Geometry check sheet. Reference: the model listing, model coordinates, mm. Give positions to 0.01 mm unless a question says otherwise; leave off trailing zeros. Order: outer loops, then holes, each group sorted by start corner. A loop starts at its lowest first (then second) coordinate and runs counter-clockwise, first axis right, second up. Notation, with made-up numbers: M -4,-32.5 L 11,-32.5 A32 cw 11,-1.5 Z; hole C 0.25,-31.75 d2. An arc over 180 degrees is marked long. Put each result on its own line as item: value. Start each with the question number.
Q1. Section check A-A on x = 0. Record the cut outline in (y, z) (3 decimals).
Q2. Section check C-C on x = -36. Record the cut outline in (y, z) (3 decimals).
Q3. Material ranges on L1, parallel to Z at x = -39, y = -72 (3 decimals); L2, parallel to Y at x = 17, z = -2; L3, parallel to Y at x = -4, z = -1.75, recorded low to high.
Q4. Section check D-D on y = -52. Record the cut outline in (x, z) (3 decimals), then the cut area to 3 significant figures.
Q5. Go/stop test with flat-tipped pins: pin 1 (2 mm diameter, centred on y = 0, z = 0, fed in from +X); pin 2 (3 mm diameter, centred on y = 72, z = 0, fed in from -X). Record where each tip stops, or that it passes through.
Q6. Section check B-B on y = 23.5. Record the cut outline in (x, z) (3 decimals), then the cut area to 3 significant figures.
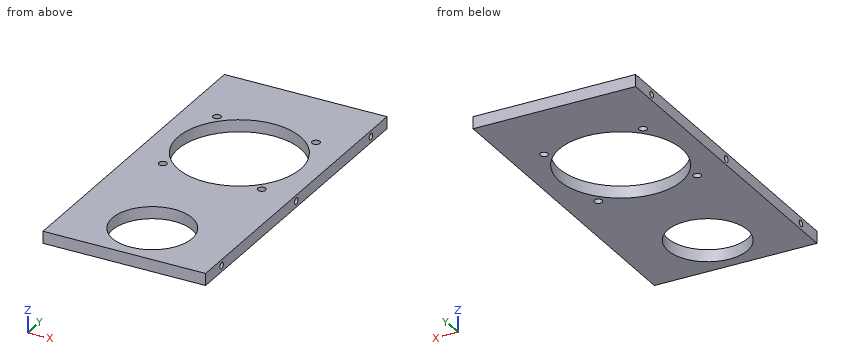
```python
from build123d import *

# Parameters (mm, degrees)
SKETCH1_W           = 86
SKETCH1_H           = 175
BOSS_EXTRUDE1_DEPTH = 3.175
SKETCH3_R           = 1.65
CUT_EXTRUDE1_DEPTH  = 10
SKETCH4_R           = 32.5
CUT_EXTRUDE2_DEPTH  = 98.701445742
SKETCH4_3_R         = 2.1
CUT_EXTRUDE3_DEPTH  = 98.701445742
SKETCH7_R           = 21.1
CUT_EXTRUDE4_DEPTH  = 98.701445742


with BuildPart() as part:
    # Sketch1 → Boss-Extrude1 (new, symmetric)
    with BuildSketch(Plane.XY):
        Rectangle(SKETCH1_W, SKETCH1_H)
    extrude(amount=BOSS_EXTRUDE1_DEPTH, both=True)

    # Sketch3 → Cut-Extrude1 (cut)
    with BuildSketch(Plane.ZY.offset(43)):
        with Locations(Location((0, 72, 0), (0, 0, 270))):
            Circle(SKETCH3_R)
        with Locations(Location((0, 0, 0), (0, 0, 270))):
            Circle(SKETCH3_R)
        with Locations(Location((0, -72, 0), (0, 0, 270))):
            Circle(SKETCH3_R)
    cut_extrude1 = extrude(amount=-CUT_EXTRUDE1_DEPTH, mode=Mode.SUBTRACT)

    # Mirror1: Cut-Extrude1 across plane
    add(cut_extrude1.mirror(Plane(origin=(0, 0, 0), x_dir=(0, 0, 1), z_dir=(1, 0, 0))), mode=Mode.SUBTRACT)

    # Sketch4 → Cut-Extrude2 (cut, through all)
    with BuildSketch(Plane.XY.offset(3.175)):
        with Locations((0, 23.5)):
            Circle(SKETCH4_R)
    extrude(amount=-CUT_EXTRUDE2_DEPTH, mode=Mode.SUBTRACT)

    # Sketch4_3 → Cut-Extrude3 (cut, through all)
    with BuildSketch(Plane.XY.offset(3.175)):
        with Locations((-26.162950904, 49.662950904)):
            Circle(SKETCH4_3_R)
        with Locations((26.162950904, 49.662950904)):
            Circle(SKETCH4_3_R)
        with Locations((26.162950904, -2.662950904)):
            Circle(SKETCH4_3_R)
        with Locations((-26.162950904, -2.662950904)):
            Circle(SKETCH4_3_R)
    extrude(amount=-CUT_EXTRUDE3_DEPTH, mode=Mode.SUBTRACT)

    # Sketch7 → Cut-Extrude4 (cut, through all)
    with BuildSketch(Plane.XY.offset(3.175)):
        with Locations((0, -60.5)):
            Circle(SKETCH7_R)
    extrude(amount=-CUT_EXTRUDE4_DEPTH, mode=Mode.SUBTRACT)


solid = part.part
```
Results found:
1. outline: M -87.5,-3.175 L -81.6,-3.175 L -81.6,3.175 L -87.5,3.175 Z; M -39.4,-3.175 L -9,-3.175 L -9,3.175 L -39.4,3.175 Z; M 56,-3.175 L 87.5,-3.175 L 87.5,3.175 L 56,3.175 Z
2. outline: M -87.5,-3.175 L 87.5,-3.175 L 87.5,3.175 L -87.5,3.175 Z; hole C -72,0 d3.3; hole C 0,0 d3.3; hole C 72,0 d3.3
3. L1: z = -3.175 to -1.65, 1.65 to 3.175
3. L2: y = -87.5 to -73, -48 to -4.2, 51.2 to 87.5
3. L3: y = -87.5 to -81.22, -39.78 to -8.75, 55.75 to 87.5
4. outline: M -43,-3.175 L -19.312,-3.175 L -19.312,3.175 L -43,3.175 Z; M 19.312,-3.175 L 43,-3.175 L 43,3.175 L 19.312,3.175 Z
4. area: 301 mm^2
5. pin 1: stops at x = 33
5. pin 2: stops at x = -33
6. outline: M -43,-3.175 L -32.5,-3.175 L -32.5,3.175 L -43,3.175 Z; M 32.5,-3.175 L 43,-3.175 L 43,3.175 L 32.5,3.175 Z
6. area: 133 mm^2
